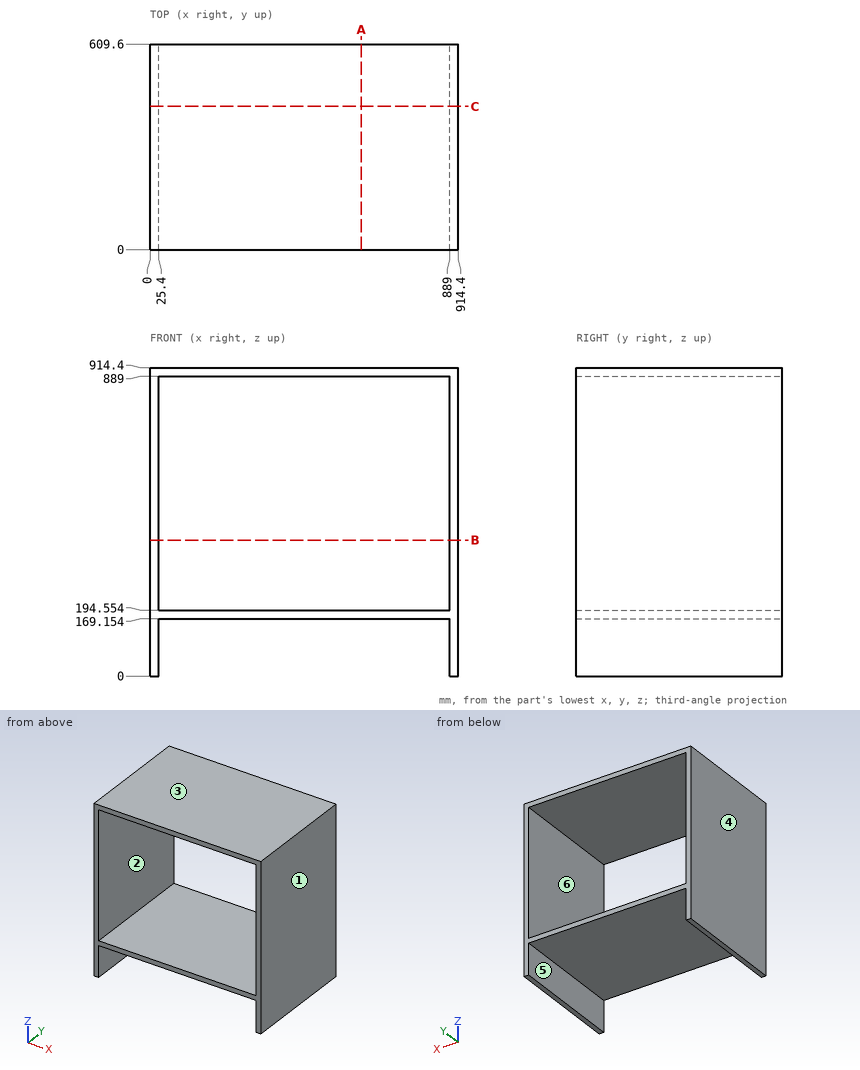
For this review, use the dimensioned drawing (mm, ordinates from the lowest corner) and the shaded views. A direction names the side the tool comes from. Give positions to 0.01 mm unless a question says otherwise; leave off trailing zeros. Order: outer loops, then holes, each group sorted by start corner. A loop starts at its lowest first (then second) coordinate and runs counter-clockwise, first axis right, second up. Notation, with made-up numbers: (36.25, 47) - (51.25, 47) arc R26 ccw to (51.25, 69) - close; hole circle Ø11 at (-38.75, 72). An arc over 180 degrees is marked (long way). Use a Markdown table: item, result. Add a question column.
(1) Mouldability with a two-part tool opening along X and no side actions: class the marked faces 1, 2 and 3 as +X half, -X half, draft (parallel to the pull), parting line (faces both ways), or undercut.
(2) Wall thickness on probe 1 along X at (y, z) = (416, 652); probe 2 along Z at (x, y) = (446.5, 167): over which ranges is each line inside the solid? List them lowest first. Write a range as [from, to].
(3) Add section B-B on z = 403. Give the boundary of the cut face in (x, y), then the cut area to 3 significant figures.
(4) Add section A-A on x = 626.5. Give the boundary of the cut face in (y, z), then the cut area to 3 significant figures.
(5) Clearance check with a flat-ended pin moving along its axis: P1, Ø10, axis at x = 343.5, y = 496, coming from the -Z side. State where the tip first meets the part, or that it passes through.
(6) Machinability: for the marked faces 4, 5 and 6, which of the approach directions +Z, -Z, +X, -X, +Y, -Y give a long, thin tool a straight path to every point of the face, cutting with its end or side? Answer none if there is none.
(7) Add section C-C on y = 425. Give the boundary of the cut face in (x, z), then the cut area to 3 significant figures.
Report:
| question | item | result |
|---|---|---|
| 1 | face 1 | +X half |
| 1 | face 2 | undercut |
| 1 | face 3 | draft |
| 2 | probe 1 | x = [0, 25.4], [889, 914.4] |
| 2 | probe 2 | z = [169.15, 194.55], [889, 914.4] |
| 3 | outline | (0, 0) - (25.4, 0) - (25.4, 609.6) - (0, 609.6) - close; (889, 0) - (914.4, 0) - (914.4, 609.6) - (889, 609.6) - close |
| 3 | area | 31,000 mm² |
| 4 | outline | (0, 169.15) - (609.6, 169.15) - (609.6, 194.55) - (0, 194.55) - close; (0, 889) - (609.6, 889) - (609.6, 914.4) - (0, 914.4) - close |
| 4 | area | 31,000 mm² |
| 5 | P1 | stops at z = 169.15 |
| 6 | face 4 | +Z, -Z, -X, +Y, -Y |
| 6 | face 5 | -Z, +Y, -Y |
| 6 | face 6 | +Y, -Y |
| 7 | outline | (0, 0) - (25.4, 0) - (25.4, 169.15) - (889, 169.15) - (889, 0) - (914.4, 0) - (914.4, 914.4) - (0, 914.4) - close; hole (25.4, 194.55) - (889, 194.55) - (889, 889) - (25.4, 889) - close |
| 7 | area | 90,300 mm² |
